```python
from build123d import *

# Parameters (mm, degrees)
SPHERE_ANGLE         = 180
SPHERE_ROLL_ANGLE    = 90
CYLINDER001_R        = 2
CYLINDER001_DEPTH    = 10
CYLINDER_R           = 5
CYLINDER_DEPTH       = 92
CYLINDER_PITCH_ANGLE = 90


with BuildPart() as sphere:
    # Sphere → Sphere (revolve)
    with BuildSketch(Plane.XZ):
        with BuildLine():
            ThreePointArc((0, -3.5), (3.5, 0), (0, 3.5))
            Line((0, 3.5), (0, -3.5))
        make_face()
    revolve(axis=Axis((0, 0, 0), (0, 0, 1)), revolution_arc=SPHERE_ANGLE)


with BuildPart() as sphere_1:
    # Sphere roll: moved
    add(sphere.part.rotate(Axis((0, 0, 0), (1, 0, 0)), SPHERE_ROLL_ANGLE))


with BuildPart() as sphere_2:
    # Sphere placement: moved
    add(sphere_1.part.moved(Location((55, 0, 19))))


with BuildPart() as cylinder001:
    # Cylinder001 → Cylinder001 (new body)
    with BuildSketch(Plane(origin=(55, 0, 9), x_dir=(1, 0, 0), z_dir=(0, 0, 1))):
        Circle(CYLINDER001_R)
    extrude(amount=CYLINDER001_DEPTH)


with BuildPart() as fusion001:
    # Cylinder → Cylinder (new body)
    with BuildSketch(Plane.XY):
        Circle(CYLINDER_R)
    extrude(amount=CYLINDER_DEPTH)


with BuildPart() as fusion001_1:
    # Cylinder pitch: moved
    add(fusion001.part.rotate(Axis((0, 0, 0), (0, 1, 0)), CYLINDER_PITCH_ANGLE))


with BuildPart() as fusion001_2:
    # Cylinder placement: moved
    add(fusion001_1.part.moved(Location((0, 0, 5))))

    # Fusion: union Cylinder001
    add(cylinder001.part)

    # Fusion001: union Sphere
    add(sphere_2.part)


solid = fusion001_2.part
```
Geometry: final body of the model. Coordinates: model frame, mm. Round coordinates to 2 decimals unless told otherwise and drop trailing zeros. Loops run counter-clockwise (first coordinate to the right, second up) from the corner with the lowest first, then second, coordinate; pieces in that order, holes last. Notation, with made-up numbers: (62.5, 16.25) -> (71.5, 16.25) arc R9 cw to (71.5, 21.25) -> close; hole circle Ø8 at (30, 52.25). An arc over 180 degrees is marked (long way). Write each question's results on one line, items separated by ' | '.
Item 1: Pull-direction query (Z, two-part tool) for faces 1 (the face through (92, 0, 5)), 2 (the face through (57, 2, 19)), 3 (the face through (53, 0, 14)); classes: pulls with the +Z half, pulls with the -Z half, needs draft (parallel to the pull), parting line crosses it, or undercut.
Answers below:
face 1: needs draft | face 2: undercut | face 3: undercut
Item 2: Cut plane D-D on z = 20.5. Return the cut outline in (x, y).
Answers below:
outline: circle Ø6.32 at (55, 0)
Item 3: Cut plane A-A on y = 0. Return the cut outline in (x, z), and give its area (3 significant figures).
Answers below:
outline: (0, 0) -> (92, 0) -> (92, 10) -> (57, 10) -> (57, 19) -> (58.5, 19) arc R3.5 ccw to (51.5, 19) -> (53, 19) -> (53, 10) -> (0, 10) -> close | area: 975 mm²
Item 4: Cut plane B-B on x = 55. Return the cut outline in (y, z).
Answers below:
outline: (-3.5, 19) -> (-2, 19) -> (-2, 9.58) arc R5 ccw (long way) to (2, 9.58) -> (2, 19) -> (3.5, 19) arc R3.5 ccw to start
Item 5: Pin query (flat end, axial travel): pin 1 Ø8 at (x, z) = (41.5, 15.5) entering from +Y; pin 2 Ø6 at (x, y) = (53.5, 3) entering from +Z; pin 3 Ø5 at (x, y) = (43.5, 1) entering from +Z; pin 4 Ø2 at (x, z) = (19, 6.5) entering from +Y. Return the tip coordinate at first contact, or that it passes through.
Answers below:
pin 1: passes through | pin 2: stops at z = 22.48 | pin 3: stops at z = 10 | pin 4: stops at y = 4.97
Item 6: Cut plane C-C on z = 11.25. Return the cut outline in (x, y), and give its area (3 significant figures).
Answers below:
outline: circle Ø4 at (55, 0) | area: 12.6 mm²
Item 7: Line query: probe 1 along Z at (x, y) = (55.5, 2.5); probe 2 along Z at (x, y) = (25, -2.5); probe 3 along Y at (x, z) = (52, 2.25). Output: solid intervals per line, ascending. Write a range as [from, to].
Answers below:
probe 1: z = [0.67, 9.33], [19, 21.4] | probe 2: z = [0.67, 9.33] | probe 3: y = [-4.18, 4.18]
